```python
from build123d import *

# Parameters (mm, degrees)
F1_DEPTH = 5
F2_DEPTH = 20
F4_DEPTH = 37.6
F5_SIZE  = 2
F6_R     = 5


# Not quite as in the source:
# - a pattern or mirror of a feature is missing from the dataset's text; its kind, count and spacing are read off the source's solid


with BuildPart() as f1:
    # F0 (on Top) → F1 (new body)
    with BuildSketch(Plane.XY):
        with BuildLine():
            Line((11.2583302492, 6.5), (0, 0))
            Line((0, 0), (28.8675134595, 0))
            Line((28.8675134595, 0), (28.8675134595, 12.6666666667))
            ThreePointArc((28.8675134595, 12.6666666667), (26.8675134595, 13.2025650515), (25.4034118443, 14.6666666667))
            Line((25.4034118443, 14.6666666667), (14.7224318643, 8.5))
            ThreePointArc((14.7224318643, 8.5), (14.9222327093, 8.0176380902), (14.9903810568, 7.5))
            ThreePointArc((14.9903810568, 7.5), (13.508019147, 5.5681483474), (11.2583302492, 6.5))
        make_face()
        with BuildLine():
            Line((14.4337567297, 25), (0, 0))
            Line((0, 0), (11.2583302492, 6.5))
            ThreePointArc((11.2583302492, 6.5), (11.9903810568, 9.2320508076), (14.7224318643, 8.5))
            Line((14.7224318643, 8.5), (25.4034118443, 14.6666666667))
            ThreePointArc((25.4034118443, 14.6666666667), (24.8675134595, 16.6666666667), (25.4034118443, 18.6666666667))
            Line((25.4034118443, 18.6666666667), (14.4337567297, 25))
        make_face()
        with BuildLine():
            Line((28.8675134595, 12.6666666667), (28.8675134595, 0))
            Line((28.8675134595, 0), (57.735026919, 0))
            Line((57.735026919, 0), (46.4766966698, 6.5))
            ThreePointArc((46.4766966698, 6.5), (43.7446458622, 5.7679491924), (43.0125950546, 8.5))
            Line((43.0125950546, 8.5), (32.3316150746, 14.6666666667))
            ThreePointArc((32.3316150746, 14.6666666667), (30.8675134595, 13.2025650515), (28.8675134595, 12.6666666667))
        make_face()
        with BuildLine():
            ThreePointArc((28.8675134595, 20.6666666667), (26.8675134595, 20.1307682818), (25.4034118443, 18.6666666667))
            Line((25.4034118443, 18.6666666667), (28.8675134595, 16.6666666667))
            Line((28.8675134595, 16.6666666667), (28.8675134595, 20.6666666667))
        make_face()
        with BuildLine():
            Line((28.8675134595, 16.6666666667), (25.4034118443, 18.6666666667))
            ThreePointArc((25.4034118443, 18.6666666667), (24.8675134595, 16.6666666667), (25.4034118443, 14.6666666667))
            Line((25.4034118443, 14.6666666667), (28.8675134595, 16.6666666667))
        make_face()
        with BuildLine():
            Line((46.4766966698, 6.5), (57.735026919, 0))
            Line((57.735026919, 0), (43.3012701892, 25))
            Line((43.3012701892, 25), (32.3316150746, 18.6666666667))
            ThreePointArc((32.3316150746, 18.6666666667), (32.7312167646, 17.7019428471), (32.8675134595, 16.6666666667))
            ThreePointArc((32.8675134595, 16.6666666667), (32.7312167646, 15.6313904863), (32.3316150746, 14.6666666667))
            Line((32.3316150746, 14.6666666667), (43.0125950546, 8.5))
            ThreePointArc((43.0125950546, 8.5), (45.2622839524, 9.4318516526), (46.7446458622, 7.5))
            ThreePointArc((46.7446458622, 7.5), (46.6764975148, 6.9823619098), (46.4766966698, 6.5))
        make_face()
        with BuildLine():
            ThreePointArc((25.4034118443, 14.6666666667), (26.8675134595, 13.2025650515), (28.8675134595, 12.6666666667))
            Line((28.8675134595, 12.6666666667), (28.8675134595, 16.6666666667))
            Line((28.8675134595, 16.6666666667), (25.4034118443, 14.6666666667))
        make_face()
        with BuildLine():
            Line((28.8675134595, 16.6666666667), (28.8675134595, 12.6666666667))
            ThreePointArc((28.8675134595, 12.6666666667), (30.8675134595, 13.2025650515), (32.3316150746, 14.6666666667))
            Line((32.3316150746, 14.6666666667), (28.8675134595, 16.6666666667))
        make_face()
        with BuildLine():
            Line((28.8675134595, 20.6666666667), (28.8675134595, 16.6666666667))
            Line((28.8675134595, 16.6666666667), (32.3316150746, 18.6666666667))
            ThreePointArc((32.3316150746, 18.6666666667), (30.8675134595, 20.1307682818), (28.8675134595, 20.6666666667))
        make_face()
        with BuildLine():
            Line((32.3316150746, 18.6666666667), (28.8675134595, 16.6666666667))
            Line((28.8675134595, 16.6666666667), (32.3316150746, 14.6666666667))
            ThreePointArc((32.3316150746, 14.6666666667), (32.7312167646, 15.6313904863), (32.8675134595, 16.6666666667))
            ThreePointArc((32.8675134595, 16.6666666667), (32.7312167646, 17.7019428471), (32.3316150746, 18.6666666667))
        make_face()
    extrude(amount=F1_DEPTH)

    # F1_copies: F1 across plane


with BuildPart() as f1_1:
    add(f1.part)
    add(f1.part.mirror(Plane(origin=(0, 0, 0), x_dir=(0.8660254038, 0.5, 0), z_dir=(-0.5, 0.8660254038, 0))))

    # F0 (on Top) → F2 (join)
    with BuildSketch(Plane.XY):
        with BuildLine():
            Line((32.3316150746, 18.6666666667), (28.8675134595, 16.6666666667))
            Line((28.8675134595, 16.6666666667), (32.3316150746, 14.6666666667))
            ThreePointArc((32.3316150746, 14.6666666667), (32.7312167646, 15.6313904863), (32.8675134595, 16.6666666667))
            ThreePointArc((32.8675134595, 16.6666666667), (32.7312167646, 17.7019428471), (32.3316150746, 18.6666666667))
        make_face()
        with BuildLine():
            Line((28.8675134595, 20.6666666667), (28.8675134595, 16.6666666667))
            Line((28.8675134595, 16.6666666667), (32.3316150746, 18.6666666667))
            ThreePointArc((32.3316150746, 18.6666666667), (30.8675134595, 20.1307682818), (28.8675134595, 20.6666666667))
        make_face()
        with BuildLine():
            ThreePointArc((28.8675134595, 20.6666666667), (26.8675134595, 20.1307682818), (25.4034118443, 18.6666666667))
            Line((25.4034118443, 18.6666666667), (28.8675134595, 16.6666666667))
            Line((28.8675134595, 16.6666666667), (28.8675134595, 20.6666666667))
        make_face()
        with BuildLine():
            Line((28.8675134595, 16.6666666667), (25.4034118443, 18.6666666667))
            ThreePointArc((25.4034118443, 18.6666666667), (24.8675134595, 16.6666666667), (25.4034118443, 14.6666666667))
            Line((25.4034118443, 14.6666666667), (28.8675134595, 16.6666666667))
        make_face()
        with BuildLine():
            ThreePointArc((25.4034118443, 14.6666666667), (26.8675134595, 13.2025650515), (28.8675134595, 12.6666666667))
            Line((28.8675134595, 12.6666666667), (28.8675134595, 16.6666666667))
            Line((28.8675134595, 16.6666666667), (25.4034118443, 14.6666666667))
        make_face()
        with BuildLine():
            Line((28.8675134595, 16.6666666667), (28.8675134595, 12.6666666667))
            ThreePointArc((28.8675134595, 12.6666666667), (30.8675134595, 13.2025650515), (32.3316150746, 14.6666666667))
            Line((32.3316150746, 14.6666666667), (28.8675134595, 16.6666666667))
        make_face()
    extrude(amount=-F2_DEPTH)

    # F3 (on Right) → F4 (cut)
    with BuildSketch(Plane.YZ):
        with BuildLine():
            ThreePointArc((15.165, -19.25), (16.665, -20.75), (18.165, -19.25))
            ThreePointArc((18.165, -19.25), (16.665, -17.75), (15.165, -19.25))
        make_face()
    extrude(amount=F4_DEPTH, mode=Mode.SUBTRACT)

    # F5
    f5_edges = [f1_1.edges().sort_by_distance(p)[0] for p in [
        (10.990381, 7.5, 0),
        (28.867513, 37, 0),
        (46.476697, 6.5, 0),
    ]]
    chamfer(f5_edges, length=F5_SIZE)

    # F6
    f6_edges = [f1_1.edges().sort_by_distance(p)[0] for p in [
        (57.735027, 0, 2.5),
        (0, 0, 2.5),
        (28.867513, 50, 2.5),
    ]]
    fillet(f6_edges, radius=F6_R)


solid = f1_1.part
```
Can you work these out from the model? Positions are in its coordinate system, mm. Give positions to 0.01 mm unless a question says otherwise; leave off trailing zeros. Write each loop counter-clockwise with the first axis right and the second up, starting at its lowest first coordinate (ties: lowest second). Pieces come first, ordered by that corner, then holes. Notation, with made-up numbers: (23.25, 68.25) - (64.25, 68.25) arc R27 ccw to (64.25, 97.25) - close; hole circle Ø8 at (-11.75, 31). An arc over 180 degrees is marked (long way). Write item = value, one per line. Start each with the question number.
1. Imagine slicing it at C-C (z = -19.25). Please give me the cut outline in (x, y) (3 decimals).
2. Imagine slicing it at D-D (x = 22.5). Please give me the cut outline in (y, z).
3. Imagine slicing it at A-A (y = 35). Please give me the cut outline in (x, z).
4. For pin 1 (12 mm diameter, centred on x = 24.5, z = -14, fed in from -Y); pin 2 (10 mm diameter, centred on x = 17, y = 37, fed in from -Z); pin 3 (1.5 mm diameter, centred on y = 18.5, z = 2, fed in from +X); pin 4 (22.5 mm diameter, centred on x = 40.5, y = 24.5, fed in from -Z), each with a flat end and sliding along its axis, tell me the tip position at first contact or that it passes through.
5. Please list where these lines run through material, in increasing order: line 1 (Z direction, x = 34, y = 14.5); line 2 (Y direction, x = 30.5, z = -19.25) (3 decimals); line 3 (X direction, y = 36, z = 2.5).
6. Imagine slicing it at B-B (z = -5). Please give me the cut outline in (x, y).
Worked answers:
q1.outline = (25.159, 18.165) - (32.576, 18.165) arc R4 ccw to start; (25.16, 15.165) arc R4 ccw to (32.575, 15.165) - close
q2.outline = (0, 0) - (38.97, 0) - (38.97, 5) - (0, 5) - close
q3.outline = (20.21, 0) - (24.87, 0) - (26.87, 2) - (26.87, 5) - (20.21, 5) - close; (30.87, 2) - (32.87, 0) - (37.53, 0) - (37.53, 5) - (30.87, 5) - close
q4.pin_1 = 12.67
q4.pin_2 = 0
q4.pin_3 = 47.49
q4.pin_4 = -20
q5.line_1 = 0 to 5
q5.line_2 = 13.015 to 15.165, 18.165 to 20.318
q5.line_3 = 20.78 to 27.14, 30.6 to 36.95
q6.outline = circle Ø8 at (28.87, 16.67)
